Source: CAD feature listing. Evaluate the final solid. Frame: model axes, mm. Face numbers are marked on the shaded views. A direction names the side the tool comes from. Give positions to 0.01 mm unless a question says otherwise; leave off trailing zeros. Order: outer loops, then holes, each group sorted by start corner. A loop starts at its lowest first (then second) coordinate and runs counter-clockwise, first axis right, second up. Notation, with made-up numbers: (44.25, 42) -> (72.25, 42) arc R19 cw to (72.25, 51) -> close; hole circle Ø2 at (-18.75, -5.5). An arc over 180 degrees is marked (long way). Answer in a Markdown table with one row per item.
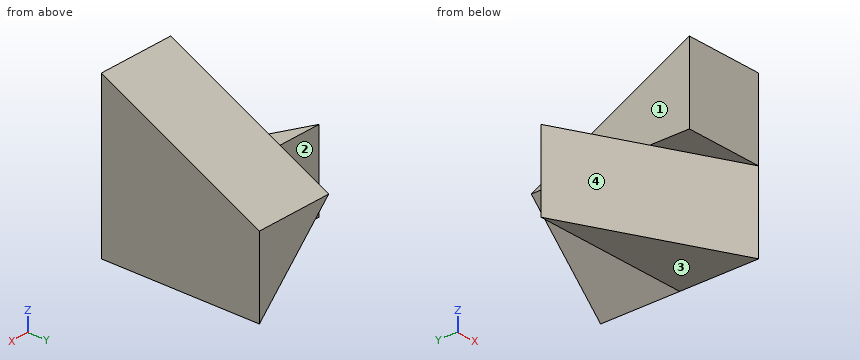
```python
from build123d import *

# Parameters (mm, degrees)
SKETCH1_W           = 40
SKETCH1_H           = 40
BOSS_EXTRUDE1_DEPTH = 40
SKETCH2_W           = 20
SKETCH2_H           = 20
CUT_EXTRUDE1_DEPTH  = 40
CUT_EXTRUDE2_DEPTH  = 40
CUT_EXTRUDE3_DEPTH  = 40
SKETCH5_W           = 20
SKETCH5_H           = 20
CUT_EXTRUDE4_DEPTH  = 40
CUT_EXTRUDE5_DEPTH  = 20
CUT_EXTRUDE13_DEPTH = 20


with BuildPart() as part:
    # Sketch1 → Boss-Extrude1 (new body)
    with BuildSketch(Plane.XY):
        with Locations((20, 20)):
            Rectangle(SKETCH1_W, SKETCH1_H)
    extrude(amount=BOSS_EXTRUDE1_DEPTH)

    # Sketch2 → Cut-Extrude1 (cut)
    with BuildSketch(Plane.XY.offset(40)):
        with Locations((10, 30)):
            Rectangle(SKETCH2_W, SKETCH2_H)
    extrude(amount=-CUT_EXTRUDE1_DEPTH, mode=Mode.SUBTRACT)

    # Sketch3 → Cut-Extrude2 (cut)
    with BuildSketch(Plane.XY.offset(40)):
        Polygon((0, 0), (20, 0), (20, 10), (0, 20), align=None)
    extrude(amount=-CUT_EXTRUDE2_DEPTH, mode=Mode.SUBTRACT)

    # Sketch4 → Cut-Extrude3 (cut)
    with BuildSketch(Plane(origin=(40, 0, 0), x_dir=(0, 0, -1), z_dir=(1, 0, 0))):
        Polygon((-40, 0), (-20, 40), (-40, 40), align=None)
    extrude(amount=-CUT_EXTRUDE3_DEPTH, mode=Mode.SUBTRACT)

    # Sketch5 → Cut-Extrude4 (cut)
    with BuildSketch(Plane.XZ):
        with Locations((10, 30)):
            Rectangle(SKETCH5_W, SKETCH5_H)
    extrude(amount=-CUT_EXTRUDE4_DEPTH, mode=Mode.SUBTRACT)

    # Sketch6 → Cut-Extrude5 (cut)
    with BuildSketch(Plane(origin=(0, 0, 0), x_dir=(-1, 0, 0), z_dir=(0, 0, -1))):
        Polygon((-20, 10), (-40, 0), (-20, 0), align=None)
    extrude(amount=-CUT_EXTRUDE5_DEPTH, mode=Mode.SUBTRACT)

    # Sketch9 → Cut-Extrude13 (cut)
    with BuildSketch(Plane(origin=(0, 40, 0), x_dir=(1, 0, 0), z_dir=(0, 1, 0))):
        Polygon((20, -20), (40, 0), (20, 0), align=None)
    extrude(amount=-CUT_EXTRUDE13_DEPTH, mode=Mode.SUBTRACT)


solid = part.part
```
(1) Access query for the marked faces 1, 2, 3 and 4. Directions: +Z, -Z, +X, -X, +Y, -Y. A direction counts if a zero-diameter tool reaches every point of the face in a straight line with its end or side. Return the directions, or none.
A:
| item | result |
|---|---|
| face 1 | +Z, -X, +Y, -Y |
| face 2 | -Z, -X, +Y |
| face 3 | -Z, +X, -X, +Y, -Y |
| face 4 | -Z, -X, -Y |
(2) Section query B-B (z = 10). Return the cut outline in (x, y), plus the area to 3 significant figures.
A:
| item | result |
|---|---|
| outline | (0, 20) -> (40, 0) -> (40, 40) -> (30, 40) -> (30, 20) -> close |
| area | 600 mm^2 |
(3) Ray query, probe 1 along X at (y, z) = (5, 23.5); probe 2 along Z at (x, y) = (18.5, 18.5); probe 3 along X at (y, z) = (24.5, 11). Return the intervals inside material, ascending.
A:
| item | result |
|---|---|
| probe 1 | x = 20 to 40 |
| probe 2 | z = 0 to 20 |
| probe 3 | x = 29 to 40 |
(4) First-contact query: pin 1 Ø8 at (x, y) = (33.5, 5.5) entering from -Z; pin 2 Ø1.5 at (x, y) = (10.5, 21.5) entering from +Z; pin 3 Ø12 at (x, y) = (20.5, 11) entering from +Z; pin 4 Ø1.5 at (y, z) = (15, 24) entering from -X. Flat tips, straight axial feed; report the tip coordinate or a pass-through.
A:
| item | result |
|---|---|
| pin 1 | stops at z = 0 |
| pin 2 | passes through |
| pin 3 | stops at z = 37.5 |
| pin 4 | stops at x = 20 |
(5) Section query A-A (x = 22). Return the cut outline in (y, z), plus the area to 3 significant figures.
A:
| item | result |
|---|---|
| outline | (0, 20) -> (9, 20) -> (9, 0) -> (20, 0) -> (20, 18) -> (40, 18) -> (40, 20) -> (0, 40) -> close |
| area | 660 mm^2 |
(6) Section query C-C (y = 5.5). Return the cut outline in (x, z).
A:
| item | result |
|---|---|
| outline | (20, 20) -> (29, 20) -> (29, 0) -> (40, 0) -> (40, 37.25) -> (20, 37.25) -> close |
(7) Section query D-D (x = 27). Return the cut outline in (y, z).
A:
| item | result |
|---|---|
| outline | (0, 20) -> (6.5, 20) -> (6.5, 0) -> (20, 0) -> (20, 13) -> (40, 13) -> (40, 20) -> (0, 40) -> close |
